Design review of the part built by this model. Coordinates are the model's own, in mm. A direction names the side the tool comes from. Give positions to 0.01 mm unless a question says otherwise; leave off trailing zeros. Order: outer loops, then holes, each group sorted by start corner. A loop starts at its lowest first (then second) coordinate and runs counter-clockwise, first axis right, second up. Notation, with made-up numbers: (13.5, 73.5) -> (26.5, 73.5) arc R27 cw to (26.5, 96.5) -> close; hole circle Ø2 at (88.25, 69). An arc over 180 degrees is marked (long way). One line per item, written item: value. Start each with the question number.
1) Tool access review of faces 1 (the face through (-6.15, 18, 3)), 2 (the face through (26.6, 24.14, 3.22)): name each direction out of +Z, -Z, +X, -X, +Y, -Y from which nothing blocks a thin tool from reaching the whole face with its end or side.
2) Consider section D-D (z = 3). State how many separate pieces and enclosed holes the cut face has, plus the area to 3 significant figures.
3) Consider section B-B (x = 0). State the section outline as (y, z) points (3 decimals), plus the area to 3 significant figures.
4) Consider section A-A (y = 0). State the section outline as (x, z) points (3 decimals), plus the area to 3 significant figures.
5) Consider section C-C (y = -19). State the section outline as (x, z) points.
6) Wall thickness on line 1 along Y through (x, z) = (0, 2) (3 decimals); line 2 along X through (y, z) = (-18, 6); line 3 along Y through (x, z) = (-9, 6.25) (3 decimals): over which ranges is each line inside the solid? List them lowest first. Write a range as from..to.
7) The part is to be moulded in two halves that separate along X. For faces 3 (the face through (0, 6, 0)), 4 (the face through (-26.64, 24.1, 3.22)), 5 (the face through (23.97, -20.07, 3.22)), say which applies: released by +X, released by -X, zero draft, split by the parting line, or undercut.
8) For pin 1 (3.5 mm diameter, centred on x = 13.755, y = 0, fed in from +Z); pin 2 (6 mm diameter, centred on x = 0, y = 0, fed in from -Z), all flat-tipped, find the tip position at first contact; note any pin that passes through.
from build123d import *

# Parameters (mm, degrees)
F0_W     = 12.7
F0_H     = 6.35
F1_DEPTH = 6.35
F2_R     = 3
F3_D     = 5
F4_D     = 4
F5_D     = 2


with BuildPart() as f1:
    # F0 (on Top) → F1 (new body)
    with BuildSketch(Plane.XY):
        Polygon((0, 25), (-27.5, 25), (-27.5, -25), (27.5, -25), (27.5, 25), align=None)
        with Locations((-12.5, -18.25)):
            Rectangle(F0_W, F0_H, mode=Mode.SUBTRACT)
        with Locations((12.5, -18.25)):
            Rectangle(F0_W, F0_H, mode=Mode.SUBTRACT)
        with Locations((-12.5, 18.25)):
            Rectangle(F0_W, F0_H, mode=Mode.SUBTRACT)
        with Locations((12.5, 18.25)):
            Rectangle(F0_W, F0_H, mode=Mode.SUBTRACT)
    extrude(amount=F1_DEPTH)

    # F2
    f2_edges = [f1.edges().sort_by_distance(p)[0] for p in [
        (27.5, -25, 3.175),
        (27.5, 25, 3.175),
        (-27.5, -25, 3.175),
        (-27.5, 25, 3.175),
    ]]
    fillet(f2_edges, radius=F2_R)

    # F3 (through all)
    with Locations(Plane(origin=(0, 0, 0), x_dir=(1, 0, 0), z_dir=(0, 0, -1))):
        with Locations((0, 0)):
            Hole(F3_D / 2)

    # F4 (through all)
    with Locations(Plane(origin=(0, 0, 0), x_dir=(1, 0, 0), z_dir=(0, 0, -1))):
        with Locations((-13.755, 0), (0, -13.755), (13.755, 0), (0, 13.755)):
            Hole(F4_D / 2)

    # F5 (through all)
    with Locations(Plane(origin=(0, 0, 0), x_dir=(1, 0, 0), z_dir=(0, 0, -1))):
        with Locations((-23.175, 20.675), (23.175, 20.675), (23.175, -20.675), (-23.175, -20.675)):
            Hole(F5_D / 2)


solid = f1.part
Checked values:
1. face 1: +Z, -Z
1. face 2: +Z, -Z, +X, +Y
2. separate pieces: 1
2. enclosed holes: 13
2. area: 2,340 mm^2
3. outline: (-25, 0) -> (-15.755, 0) -> (-15.755, 6.35) -> (-25, 6.35) -> close; (-11.755, 0) -> (-2.5, 0) -> (-2.5, 6.35) -> (-11.755, 6.35) -> close; (2.5, 0) -> (11.755, 0) -> (11.755, 6.35) -> (2.5, 6.35) -> close; (15.755, 0) -> (25, 0) -> (25, 6.35) -> (15.755, 6.35) -> close
3. area: 235 mm^2
4. outline: (-27.5, 0) -> (-15.755, 0) -> (-15.755, 6.35) -> (-27.5, 6.35) -> close; (-11.755, 0) -> (-2.5, 0) -> (-2.5, 6.35) -> (-11.755, 6.35) -> close; (2.5, 0) -> (11.755, 0) -> (11.755, 6.35) -> (2.5, 6.35) -> close; (15.755, 0) -> (27.5, 0) -> (27.5, 6.35) -> (15.755, 6.35) -> close
4. area: 267 mm^2
5. outline: (-27.5, 0) -> (-18.85, 0) -> (-18.85, 6.35) -> (-27.5, 6.35) -> close; (-6.15, 0) -> (6.15, 0) -> (6.15, 6.35) -> (-6.15, 6.35) -> close; (18.85, 0) -> (27.5, 0) -> (27.5, 6.35) -> (18.85, 6.35) -> close
6. line 1: y = -25..-15.755, -11.755..-2.5, 2.5..11.755, 15.755..25
6. line 2: x = -27.5..-18.85, -6.15..6.15, 18.85..27.5
6. line 3: y = -25..-21.425, -15.075..15.075, 21.425..25
7. face 3: zero draft
7. face 4: released by -X
7. face 5: undercut
8. pin 1: passes through
8. pin 2: stops at z = 0
